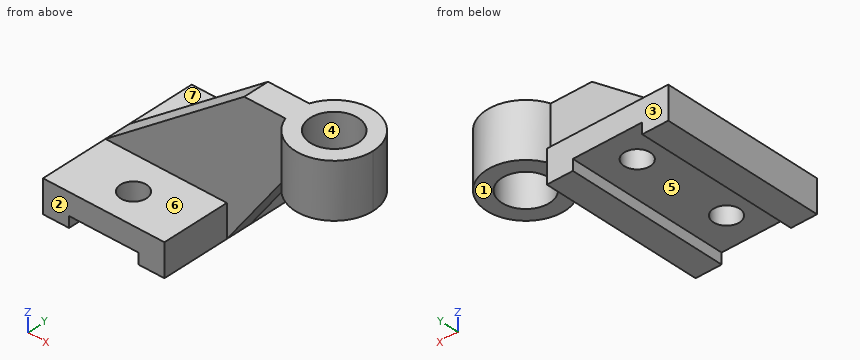
```python
from build123d import *

# Parameters (mm, degrees)
F1_DEPTH = 37.5
F0_W     = 34.9705627485
F0_H     = 25
F2_R     = 6
F2_R_2   = 11
F3_DEPTH = 63.001
F4_DEPTH = 6


with BuildPart() as f1:
    # F0 (on Front) → F1 (new body, symmetric)
    with BuildSketch(Plane.XZ):
        Polygon((0, 15), (0, 0), (12, 0), (12, 5), (44, 5), (44, 0), (56, 0), (56, 15), align=None)
    extrude(amount=F1_DEPTH, both=True)


with BuildPart() as f1b:
    # F0 (on Front) → F1, piece 2 (new body, symmetric)
    with BuildSketch(Plane.XZ):
        with Locations((100.5147186258, 50.5)):
            Rectangle(F0_W, F0_H)
    extrude(amount=F1_DEPTH, both=True)


with BuildPart() as f3_tool:
    # F2 (on face) → F3 (new body, through all)
    with BuildSketch(Plane.XY.offset(63)):
        with Locations((28, -22.5)):
            Circle(F2_R)
        with Locations((100, 0)):
            Circle(F2_R_2)
        with Locations((28, 22.5312)):
            Circle(F2_R)
        with BuildLine():
            ThreePointArc((83.0294372515, 6), (103.0438356171, 17.7407740738), (118, 0))
            Line((118, 0), (118, 37.5))
            Line((118, 37.5), (83.0294372515, 37.5))
            Line((83.0294372515, 37.5), (83.0294372515, 6))
        make_face()
        with BuildLine():
            Line((118, -37.5), (118, 0))
            ThreePointArc((118, 0), (103.0438356171, -17.7407740738), (83.0294372515, -6))
            Line((83.0294372515, -6), (83.0294372515, -37.5))
            Line((83.0294372515, -37.5), (118, -37.5))
        make_face()
    extrude(amount=-F3_DEPTH)


with BuildPart() as f1_1:
    add(f1.part)

    # F3: cut by f3_tool
    add(f3_tool.part, mode=Mode.SUBTRACT)



with BuildPart() as f1b_1:
    add(f1b.part)

    # F3: cut by f3_tool
    add(f3_tool.part, mode=Mode.SUBTRACT)


with BuildPart() as f1_2:
    add(f1_1.part)

    add(f1b_1.part)  # F4 merges F1b
    # F0 (on Front) → F4 (join, symmetric)
    with BuildSketch(Plane.XZ):
        Polygon((64, 63), (0, 15), (56, 15), (56, 0), (83.0294372515, 38), (83.0294372515, 63), (82, 63), align=None)
    extrude(amount=F4_DEPTH, both=True)


solid = f1_2.part
```
Input: part model. Units: mm. Frame: model coordinates. Face numbers are marked on the shaded views. A direction names the side the tool comes from. Give positions to 0.01 mm unless a question says otherwise; leave off trailing zeros. Order: outer loops, then holes, each group sorted by start corner. A loop starts at its lowest first (then second) coordinate and runs counter-clockwise, first axis right, second up. Notation, with made-up numbers: M 12.25,66 L 71.25,66 A6 cw 71.25,77 Z; hole C 22,21.5 d6. An arc over 180 degrees is marked long. Return JSON: item names as keys, results as strings.
Item 1: Access query for the marked faces 5, 6 and 7. Directions: +Z, -Z, +X, -X, +Y, -Y. A direction counts if a zero-diameter tool reaches every point of the face in a straight line with its end or side. Return the directions, or none.
Solutions:
{"face 5": "-Z, +Y, -Y", "face 6": "+Z, +X, -X, -Y", "face 7": "+Z, +X, -X, +Y"}
Item 2: Ray query, probe 1 along Y at (x, z) = (28, 7); probe 2 along Y at (x, z) = (100, 50); probe 3 along Y at (x, z) = (32.5, 17.5). Return the intervals inside material, ascending.
Solutions:
{"probe 1": "-37.5 to -28.5, -16.5 to 16.53, 28.53 to 37.5", "probe 2": "-18 to -11, 11 to 18", "probe 3": "-6 to 6"}
Item 3: Cut plane D-D (z = 57). Return loops of the section in (x, y).
Solutions:
{"outline": "M 56,-6 L 83.03,-6 A18 ccw long 83.03,6 L 56,6 Z; hole C 100,0 d22"}
Item 4: Cut plane B-B (y = -22.5). Return loops of the section in (x, z).
Solutions:
{"outline": "M 0,0 L 12,0 L 12,5 L 22,5 L 22,15 L 0,15 Z; M 34,5 L 44,5 L 44,0 L 56,0 L 56,15 L 34,15 Z"}
Item 5: Pull-direction query (Y, two-part tool) for the marked faces 1, 2, 3 and 4; classes: +Y half, -Y half, draft (parallel to the pull), parting line (faces both ways), or undercut.
Solutions:
{"face 1": "draft", "face 2": "-Y half", "face 3": "+Y half", "face 4": "undercut"}
Item 6: First-contact query: P1, Ø6, axis at x = 79, z = 44, coming from the -Y side; P2, Ø10, axis at x = 95.5, z = 37.5, coming from the -Y side; P3, Ø1.5, axis at x = 56, z = 20.5, coming from the +Y side. Flat tips, straight axial feed; report the tip coordinate or a pass-through.
Solutions:
{"P1": "y = -6", "P2": "y = -18", "P3": "y = 6"}
Item 7: Cut plane C-C (x = 100). Return loops of the section in (y, z).
Solutions:
{"outline": "M -18,38 L -11,38 L -11,63 L -18,63 Z; M 11,38 L 18,38 L 18,63 L 11,63 Z"}
Item 8: Cut plane A-A (x = 28). Return loops of the section in (y, z).
Solutions:
{"outline": "M -37.5,5 L -28.5,5 L -28.5,15 L -37.5,15 Z; M -16.5,5 L 16.53,5 L 16.53,15 L 6,15 L 6,36 L -6,36 L -6,15 L -16.5,15 Z; M 28.53,5 L 37.5,5 L 37.5,15 L 28.53,15 Z"}
